Read the model definition and answer for the solid it produces. Units are mm, in the model's axes. A direction names the side the tool comes from. Give positions to 0.01 mm unless a question says otherwise; leave off trailing zeros. Write each loop counter-clockwise with the first axis right and the second up, starting at its lowest first coordinate (ties: lowest second). Pieces come first, ordered by that corner, then holes. Notation, with made-up numbers: (48.25, 34.25) -> (65.25, 34.25) arc R23 cw to (65.25, 52.25) -> close; hole circle Ø9 at (78.25, 24.5). An arc over 180 degrees is marked (long way). Put each result on its own line as item: value. Start each with the question number.
from build123d import *

# Parameters (mm, degrees)
F0_W     = 25.4
F0_H     = 12.7
F1_DEPTH = 101.6
F2_DEPTH = 25.4


with BuildPart() as f1:
    # F0 (on Front) → F1 (new body)
    with BuildSketch(Plane.XZ):
        Polygon((121.018117, 50.8), (121.018117, 0), (248.018117, 0), (248.018117, 25.4), (263.420549, 25.4), (263.420549, 63.5), (238.020549, 63.5), (238.020549, 25.4), (216.686985, 25.4), (181.552551, 25.4), (171.818117, 25.4), (146.418117, 25.4), (146.418117, 38.1), (146.418117, 50.8), align=None)
        with Locations((159.118117, 31.75)):
            Rectangle(F0_W, F0_H)
    extrude(amount=F1_DEPTH)

    # F0 (on Front) → F2 (join)
    with BuildSketch(Plane.XZ):
        Polygon((121.018117, 50.8), (121.018117, 0), (248.018117, 0), (248.018117, 25.4), (263.420549, 25.4), (263.420549, 63.5), (238.020549, 63.5), (238.020549, 25.4), (216.686985, 25.4), (181.552551, 25.4), (171.818117, 25.4), (146.418117, 25.4), (146.418117, 38.1), (146.418117, 50.8), align=None)
        with Locations((159.118117, 31.75)):
            Rectangle(F0_W, F0_H)
    extrude(amount=F2_DEPTH)


solid = f1.part
1) A cutting plane is placed at C-C on x = 208. Give the vertices of the cut face in (y, z).
2) Each of these flat-tipped pins is pushed along its axis until it touches: pin 1 Ø20.5 at (x, y) = (159.5, -65.5) entering from +Z; pin 2 Ø8 at (x, y) = (139.5, -61) entering from -Z; pin 3 Ø5 at (x, y) = (210.5, -38) entering from +Z; pin 4 Ø4 at (y, z) = (-52.5, 54.5) entering from -X. Where does it stop, or does it pass through?
3) A cutting plane is placed at A-A on z = 35. Give the vertices of the cut face in (x, y).
4) For faces 1 (the face through (134, -50, 50.8)), 2 (the face through (248.018, -50, 13)), 3 (the face through (146.418, -50, 44)), 4 (the face through (263.421, -50, 44)), determine the directions among +Z, -Z, +X, -X, +Y, -Y from which every point of the face is accessible in a straight line to the end or side of a thin tool.
5) A cutting plane is placed at D-D on z = 8. Give the vertices of the cut face in (x, y).
6) Straight lines are drawn through the part: line 1 (X direction, y = -52, z = 35); line 2 (X direction, y = -22, z = 45); line 3 (Z direction, x = 172.5, y = -73). For each, find the intervals that lie inside material, in ascending order. Write a range as [from, to].
7) A cutting plane is placed at B-B on y = -85. Give the vertices of the cut face in (x, z), and give its area (3 significant figures).
Results found:
1. outline: (-101.6, 0) -> (0, 0) -> (0, 25.4) -> (-101.6, 25.4) -> close
2. pin 1: stops at z = 38.1
2. pin 2: stops at z = 0
2. pin 3: stops at z = 25.4
2. pin 4: stops at x = 238.02
3. outline: (121.02, -101.6) -> (171.82, -101.6) -> (171.82, 0) -> (121.02, 0) -> close; (238.02, -101.6) -> (263.42, -101.6) -> (263.42, 0) -> (238.02, 0) -> close
4. face 1: +Z, -X, +Y, -Y
4. face 2: -Z, +X, +Y, -Y
4. face 3: +Z, +Y, -Y
4. face 4: +Z, -Z, +X, +Y, -Y
5. outline: (121.02, -101.6) -> (248.02, -101.6) -> (248.02, 0) -> (121.02, 0) -> close
6. line 1: x = [121.02, 171.82], [238.02, 263.42]
6. line 2: x = [121.02, 146.42], [238.02, 263.42]
6. line 3: z = [0, 25.4]
7. outline: (121.02, 0) -> (248.02, 0) -> (248.02, 25.4) -> (263.42, 25.4) -> (263.42, 63.5) -> (238.02, 63.5) -> (238.02, 25.4) -> (171.82, 25.4) -> (171.82, 38.1) -> (146.42, 38.1) -> (146.42, 50.8) -> (121.02, 50.8) -> close
7. area: 5,160 mm²
